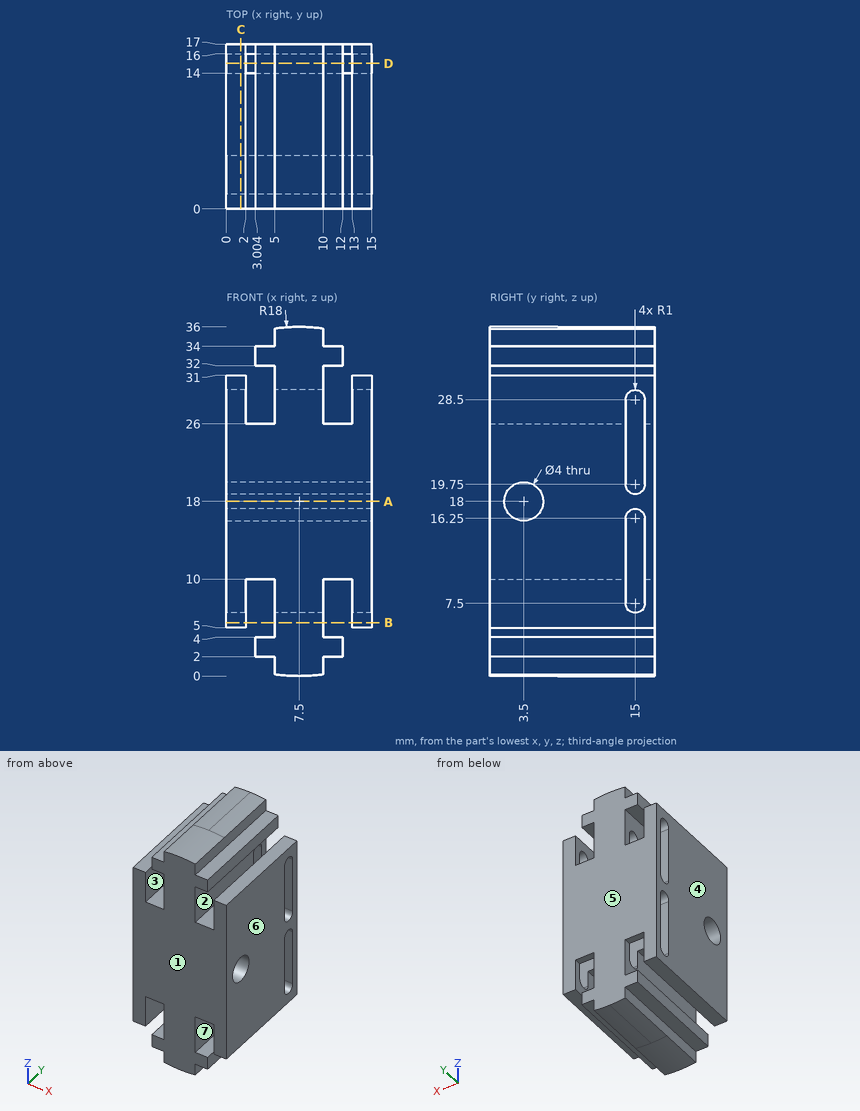
Here's the drawing with two shaded views (mm, measured from the low corner). I have some questions. A direction names the side the tool comes from. Give positions to 0.01 mm unless a question says otherwise; leave off trailing zeros. Write each loop counter-clockwise with the first axis right and the second up, starting at its lowest first coordinate (ties: lowest second). Pieces come first, ordered by that corner, then holes. Notation, with made-up numbers: (66, 32.5) - (107, 32.5) arc R23 cw to (107, 42.5) - close; hole circle Ø7 at (85.25, 87.25). An arc over 180 degrees is marked (long way). One line per item, written item: value. Start each with the question number.
Item 1: I'm going to push flat-ended pins straight in: pin 1 (1.5 mm diameter, centred on y = 9.5, z = 34.5, fed in from -X); pin 2 (2 mm diameter, centred on x = 0.5, y = 7, fed in from +Z); pin 3 (1.5 mm diameter, centred on y = 6, z = 1.5, fed in from +X). Where does each tip first touch, or does it pass through?
Item 2: Which directions (+Z, -Z, +X, -X, +Y, -Y) give clear straight access to the entire face, cutting with the end or side of a thin tool? Please do the marked faces 1, 2 and 3.
Item 3: Imagine slicing it at C-C, the plane x = 1.5. List the corners of the cut face in (y, z) for me, and give its area (3 significant figures).
Item 4: Imagine slicing it at A-A, the plane z = 18. List the corners of the cut face in (x, y) for me.
Item 5: If we mould it in two halves opening along X, with no side actions, what happens to the marked faces 4, 5, 6 and 7? For each: +X half, -X half, draft (parallel to the pull), parting line (faces both ways), or undercut.
Item 6: Imagine slicing it at D-D, the plane y = 15. Give the number of separate pieces and of enclosed holes in the cut face, and give its area (3 significant figures).
Item 7: Please list where these lines run through material, in increasing order: line 1 (Z direction, x = 4.5, y = 3.5); line 2 (X direction, y = 16.25, z = 30.5); line 3 (Z direction, x = 10.75, y = 11.5). Write a range as from..to.
Item 8: Imagine slicing it at B-B, the plane z = 5.5. List the corners of the cut face in (x, y) for me.
Geometry says:
1. pin 1: x = 3
1. pin 2: z = 31
1. pin 3: x = 12
2. face 1: +Z, -Z, +X, -X, -Y
2. face 2: +Y, -Y
2. face 3: +Z, +Y, -Y
3. outline: (0, 5) - (17, 5) - (17, 31) - (0, 31) - close; hole circle Ø4 at (3.5, 18); hole (14, 7.5) arc R1 ccw to (16, 7.5) - (16, 16.25) arc R1 ccw to (14, 16.25) - close; hole (14, 19.75) arc R1 ccw to (16, 19.75) - (16, 28.5) arc R1 ccw to (14, 28.5) - close
3. area: 388 mm^2
4. outline: (0, 0) - (15, 0) - (15, 1.5) - (0, 1.5) - close; (0, 5.5) - (15, 5.5) - (15, 17) - (0, 17) - close
5. face 4: -X half
5. face 5: draft
5. face 6: +X half
5. face 7: undercut
6. separate pieces: 7
6. enclosed holes: 0
6. area: 115 mm^2
7. line 1: 2..4, 10..16, 20..26, 32..34
7. line 2: 0..2, 5..10, 13..15
7. line 3: 2..4, 10..26, 32..34
8. outline: (0, 0) - (2, 0) - (2, 17) - (0, 17) - close; (5, 0) - (10, 0) - (10, 17) - (5, 17) - close; (13, 0) - (15, 0) - (15, 17) - (13, 17) - close
